Part model, mm, in its own coordinate system. A direction names the side the tool comes from. Coordinates: 2 decimals unless noted, no trailing zeros. Order: outer loops, then holes, each group sorted by start corner. A loop starts at its lowest first (then second) coordinate and runs counter-clockwise, first axis right, second up.
```python
from build123d import *

# Parameters (mm, degrees)
RESSALTO_EXTRUS_O1_DEPTH = 20
FILETE12_R               = 2
CHANFRO1_DEPTH           = 20
ESBO_O3_R                = 2
CORTE_EXTRUS_O1_DEPTH    = 43.712437978
ESBO_O4_R                = 2
CORTE_EXTRUS_O2_DEPTH    = 10


with BuildPart() as part:
    # Esbo_o2 → Ressalto-extrus_o1 (new body)
    with BuildSketch(Plane(origin=(0, 0, 0), x_dir=(0, 0, -1), z_dir=(1, 0, 0))):
        with BuildLine():
            Line((-18.25, 0), (18.25, 0))
            Line((18.25, 0), (28.25, 0))
            Line((28.25, 0), (28.25, 2))
            ThreePointArc((28.25, 2), (27.957106781, 2.707106781), (27.25, 3))
            Line((27.25, 3), (13.25, 3))
            ThreePointArc((13.25, 3), (12.542893219, 3.292893219), (12.25, 4))
            Line((12.25, 4), (12.25, 17))
            ThreePointArc((12.25, 17), (11.371320344, 19.121320344), (9.25, 20))
            Line((9.25, 20), (9.25, 3))
            Line((9.25, 3), (-9.25, 3))
            Line((-9.25, 3), (-9.25, 20))
            ThreePointArc((-9.25, 20), (-11.371320344, 19.121320344), (-12.25, 17))
            Line((-12.25, 17), (-12.25, 3))
            Line((-12.25, 3), (-17.25, 3))
            ThreePointArc((-17.25, 3), (-17.957106781, 2.707106781), (-18.25, 2))
            Line((-18.25, 2), (-18.25, 0))
        make_face()
    extrude(amount=RESSALTO_EXTRUS_O1_DEPTH)

    # Filete12
    filete12_edges = [part.edges().sort_by_distance(p)[0] for p in [
        (10, 3, 9.25),
        (10, 3, -9.25),
    ]]
    fillet(filete12_edges, radius=FILETE12_R)

    # Chanfro1: read off the stored shape, not the designer's step
    # Chanfro1 outline → Chanfro1 (add)
    with BuildSketch(Plane.YZ):
        Polygon((3, 12.25), (6, 12.25), (3, 15.825260778), align=None)
    extrude(amount=CHANFRO1_DEPTH)

    # Esbo_o3 → Corte-extrus_o1 (cut, through all)
    with BuildSketch(Plane(origin=(0, 9.55289202, 8.015828171), x_dir=(1, 0, 0), z_dir=(0, 0.7660444431189817, 0.6427876096865351))):
        with Locations(Location((5, -7.86090451, 0), (0, 0, 270))):
            Circle(ESBO_O3_R)
        with Locations(Location((15, -7.86090451, 0), (0, 0, 270))):
            Circle(ESBO_O3_R)
    extrude(amount=-CORTE_EXTRUS_O1_DEPTH, mode=Mode.SUBTRACT)

    # Esbo_o4 → Corte-extrus_o2 (cut)
    with BuildSketch(Plane(origin=(0, 3, 0), x_dir=(1, 0, 0), z_dir=(0, 1, 0))):
        with Locations(Location((10, 20.25, 0), (0, 0, 270))):
            Circle(ESBO_O4_R)
    extrude(amount=-CORTE_EXTRUS_O2_DEPTH, mode=Mode.SUBTRACT)


solid = part.part
```
(1) Pull direction Z, two halves, no side cores. Call faces 6 (the face through (10, 3, 0)), 7 (the face through (0, 2.5, -4.9)), 8 (the face through (9.86, 19.1, -11.39)): +Z half, -Z half, draft (parallel to the pull), parting line (faces both ways), or undercut.
(2) Tool access for faces 1 (the face through (10, 10, -12.25)), 2 (the face through (20, 2.5, -4.9)), 3 (the face through (10.14, 3.57, 8.65)), 4 (the face through (10, 3, 17)), 5 (the face through (10, 1, -28.25)): list every direction of +Z, -Z, +X, -X, +Y, -Y with a clear straight run to the whole face (end or side of a thin tool).
(3) Probe line 1 (X direction, y = 1.9, z = -20.25); line 2 (Z direction, x = 15.75, y = 12); line 3 (Y direction, x = 2.25, z = 12.5). List the from-to ranges inside material, lowest first.
(4) Slice it at A-A, the plane z = -20.25. Give the cut face in (x, y).
(5) Slice it at B-B, the plane x = 10. Give the cut face in (y, z), then the cut area to 3 significant figures.
(6) Drop flat-ended pins along their axis: pin 1 (1.5 mm diameter, centred on x = 15.5, z = -15, fed in from +Y); pin 2 (3 mm diameter, centred on y = 13.5, z = 7, fed in from +X); pin 3 (12 mm diameter, centred on x = 7.5, y = 12.5, fed in from +Z); pin 4 (4.5 mm diameter, centred on x = 15, y = 10.5, fed in from -Z). Give the stop position or say it passes through.
(7) Slice it at C-C, the plane y = 13.5. Give the cut face in (x, z).
(8) Slice it at D-D, the plane x = 1.5. Give the cut face in (y, z).
Here are the results:
1. face 6: undercut
1. face 7: draft
1. face 8: -Z half
2. face 1: -Z, +X, -X, +Y
2. face 2: +Z, -Z, +X, +Y, -Y
2. face 3: +X, -X, +Y
2. face 4: +Z, +X, -X, +Y
2. face 5: -Z, +X, -X, +Y, -Y
3. line 1: x = 0 to 8, 12 to 20
3. line 2: z = -12.25 to -9.25, 9.25 to 12.25
3. line 3: y = 0 to 5.79
4. outline: (0, 0) - (8, 0) - (8, 3) - (0, 3) - close; (12, 0) - (20, 0) - (20, 3) - (12, 3) - close
5. outline: (0, -28.25) - (2, -28.25) arc R1 ccw to (3, -27.25) - (3, -22.25) - (0, -22.25) - close; (0, -18.25) - (3, -18.25) - (3, -13.25) arc R1 cw to (4, -12.25) - (17, -12.25) arc R3 ccw to (20, -9.25) - (5, -9.25) arc R2 cw to (3, -7.25) - (3, 7.25) arc R2 cw to (5, 9.25) - (20, 9.25) arc R3 ccw to (17, 12.25) - (6, 12.25) - (3, 15.83) - (3, 17.25) arc R1 ccw to (2, 18.25) - (0, 18.25) - close
5. area: 233 mm2
6. pin 1: stops at y = 3
6. pin 2: passes through
6. pin 3: stops at z = 12.25
6. pin 4: stops at z = -12.25
7. outline: (0, -12.25) - (20, -12.25) - (20, -9.25) - (0, -9.25) - close; (0, 9.25) - (20, 9.25) - (20, 12.25) - (0, 12.25) - close
8. outline: (0, -28.25) - (2, -28.25) arc R1 ccw to (3, -27.25) - (3, -13.25) arc R1 cw to (4, -12.25) - (17, -12.25) arc R3 ccw to (20, -9.25) - (5, -9.25) arc R2 cw to (3, -7.25) - (3, 7.25) arc R2 cw to (5, 9.25) - (20, 9.25) arc R3 ccw to (17, 12.25) - (6, 12.25) - (3, 15.83) - (3, 17.25) arc R1 ccw to (2, 18.25) - (0, 18.25) - close
